The figure shows three views and two pictorial views of one solid part (mm, origin at its lowest corner). Answer the questions. A direction names the side the tool comes from. Coordinates: 2 decimals unless noted, no trailing zeros. Write each loop counter-clockwise with the first axis right and the second up, starting at its lowest first coordinate (ties: lowest second). Pieces come first, ordered by that corner, then holes.
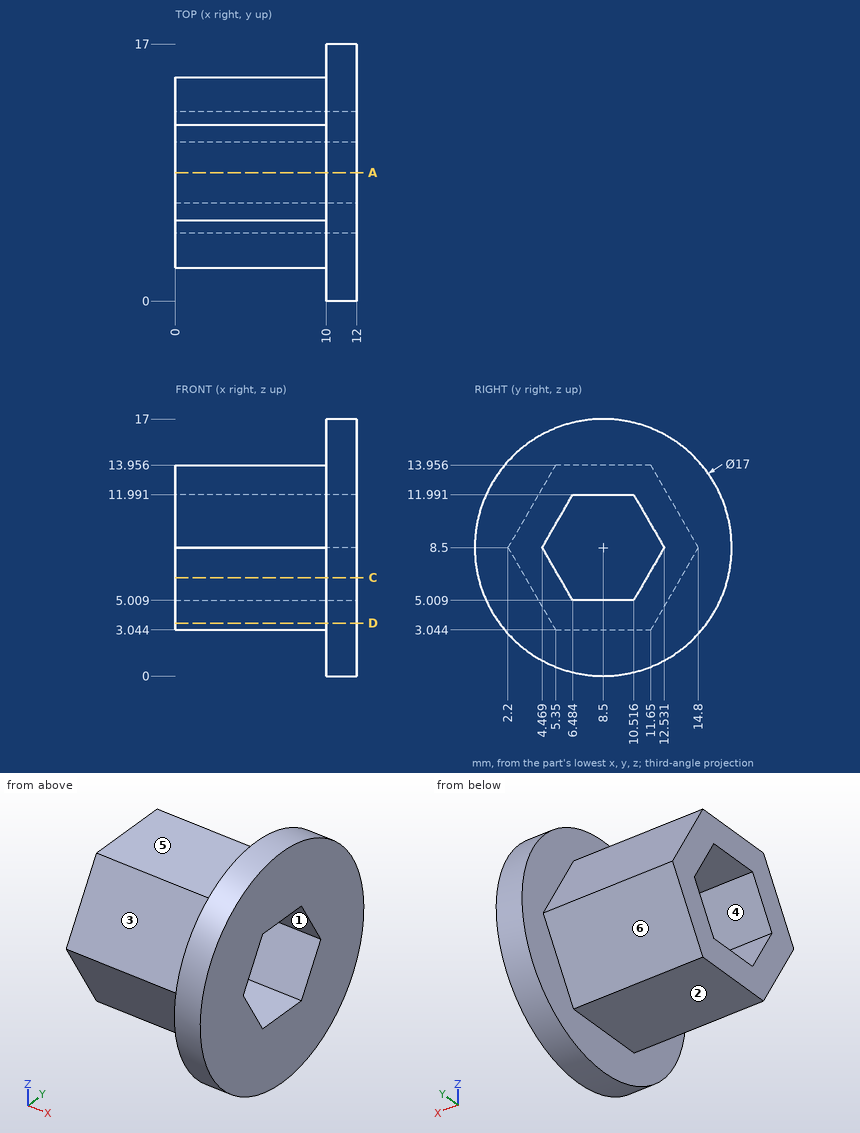
Item 1: The part is cut by section C-C (z = 6.5). Give the vertices of the cut face in (x, y) (1 decimal).
Item 2: The part is cut by section A-A (y = 8.5). Give the vertices of the cut face in (x, z).
Item 3: For the marked faces 1, 2 and 3, determine the directions among +Z, -Z, +X, -X, +Y, -Y from which every point of the face is accessible in a straight line to the end or side of a thin tool.
Item 4: Given pin 1 (4 mm diameter, centred on y = 7.5, z = 9, fed in from +X); pin 2 (4.5 mm diameter, centred on x = 5.5, y = 8, fed in from -Z); pin 3 (3 mm diameter, centred on x = 5, z = 9.5, fed in from +Y); pin 4 (3 mm diameter, centred on x = 5.5, z = 15, fed in from +Y), each flat-ended and moving along its own axis, determine where each tip first touches the part or whether it passes through.
Item 5: The part is cut by section D-D (z = 3.5). Give the vertices of the cut face in (x, y).
Item 6: Determine the mould class of the marked faces 4, 5 and 6 for opening direction Y: +Y half, -Y half, draft (parallel to the pull), parting line (faces both ways), or undercut.
Item 7: Find the intervals of material crossed by probe 1 along Z at (x, y) = (3, 9.75); probe 2 along X at (y, z) = (3.5, 2.25); probe 3 along Y at (x, z) = (1, 11.75) (1 decimal), in increasing order.
Answer:
1. outline: (0, 3.4) - (10, 3.4) - (10, 0.2) - (12, 0.2) - (12, 5.6) - (0, 5.6) - close; (0, 11.4) - (12, 11.4) - (12, 16.8) - (10, 16.8) - (10, 13.6) - (0, 13.6) - close
2. outline: (0, 3.04) - (10, 3.04) - (10, 0) - (12, 0) - (12, 5.01) - (0, 5.01) - close; (0, 11.99) - (12, 11.99) - (12, 17) - (10, 17) - (10, 13.96) - (0, 13.96) - close
3. face 1: +X, -X
3. face 2: -Z, -X, +Y, -Y
3. face 3: +Z, -X, -Y
4. pin 1: passes through
4. pin 2: stops at z = 3.04
4. pin 3: stops at y = 14.8
4. pin 4: stops at y = 11.91
5. outline: (0, 5.09) - (10, 5.09) - (10, 1.63) - (12, 1.63) - (12, 15.37) - (10, 15.37) - (10, 11.91) - (0, 11.91) - close
6. face 4: undercut
6. face 5: draft
6. face 6: +Y half
7. probe 1: z = 3.04 to 5.01, 11.99 to 13.96
7. probe 2: x = 10 to 12
7. probe 3: y = 4.1 to 6.3, 10.7 to 12.9
